from build123d import *

# Parameters (mm, degrees)
F0_R     = 9
F1_DEPTH = 5
F2_R     = 4.15
F3_DEPTH = 1.5
F4_R     = 2.65
F5_DEPTH = 5.001


with BuildPart() as f1:
    # F0 (on Front) → F1 (new body)
    with BuildSketch(Plane.XZ):
        Circle(F0_R)
    extrude(amount=F1_DEPTH)

    # F2 (on face) → F3 (cut)
    with BuildSketch(Plane(origin=(0, 0, 0), x_dir=(-1, 0, 0), z_dir=(0, 1, 0))):
        Circle(F2_R)
    extrude(amount=-F3_DEPTH, mode=Mode.SUBTRACT)

    # F4 (on face) → F5 (cut, through all)
    with BuildSketch(Plane.XZ.offset(5)):
        Circle(F4_R)
    extrude(amount=-F5_DEPTH, mode=Mode.SUBTRACT)


solid = f1.part
Source: CAD feature listing. Evaluate the final solid. Frame: model axes, mm. A direction names the side the tool comes from. Give positions to 0.01 mm unless a question says otherwise; leave off trailing zeros. Write each loop counter-clockwise with the first axis right and the second up, starting at its lowest first coordinate (ties: lowest second). Pieces come first, ordered by that corner, then holes. Notation, with made-up numbers: M 72.25,-0.5 L 105.25,-0.5 A30 cw 105.25,26.5 Z; hole C 61,-4.75 d10. An arc over 180 degrees is marked long. Return JSON: item names as keys, results as strings. Group by question number.
1) Cut plane D-D, the plane z = 6.5. Output: boundary loops of the cut face in (x, y).
2) Ray query, L1, parallel to Z at x = 0, y = -4; L2, parallel to Z at x = 0, y = -1.15; L3, parallel to X at y = -2.8, z = -0.5. Return the intervals inside material, ascending.
3) Cut plane A-A, the plane z = 0. Output: boundary loops of the cut face in (x, y), then the cut area to 3 significant figures.
4) Cut plane B-B, the plane x = 0. Output: boundary loops of the cut face in (y, z), then the cut area to 3 significant figures.
5) Cut plane C-C, the plane y = -0.5. Output: boundary loops of the cut face in (x, z).
6) Draft query along Z for faces 1 (the face through (-1.172, -2.465, 8.923)), 2 (the face through (2, 0, -4)), 3 (the face through (0, -1.5, -3)). Return one class per face: released by +Z, released by -Z, zero draft, split by the parting line, or undercut.
7) Set-up query: faces 4 (the face through (2, -5, -2)), 5 (the face through (0.9, -0.74, -4.05)). Return all of +Z, -Z, +X, -X, +Y, -Y with unobstructed straight access to the full face (end or side cutting, diameter ignored); none if empty.
8) First-contact query: pin 1 Ø5 at (x, z) = (0, 0) entering from -Y; pin 2 Ø2 at (y, z) = (-1, -5.5) entering from +X; pin 3 Ø2 at (x, z) = (-2.5, -1.5) entering from +Y; pin 4 Ø1.5 at (y, z) = (-3.5, 4.5) entering from -X. Flat tips, straight axial feed; report the tip coordinate or a pass-through.
Data:
{
 "1": {"outline": "M -6.22,-5 L 6.22,-5 L 6.22,0 L -6.22,0 Z"},
 "2": {"L1": "z = -9 to -2.65, 2.65 to 9", "L2": "z = -9 to -4.15, 4.15 to 9", "L3": "x = -8.99 to -2.6, 2.6 to 8.99"},
 "3": {"outline": "M -9,-5 L -2.65,-5 L -2.65,-1.5 L -4.15,-1.5 L -4.15,0 L -9,0 Z; M 2.65,-5 L 9,-5 L 9,0 L 4.15,0 L 4.15,-1.5 L 2.65,-1.5 Z", "area": "59.0 mm²"},
 "4": {"outline": "M -5,-9 L 0,-9 L 0,-4.15 L -1.5,-4.15 L -1.5,-2.65 L -5,-2.65 Z; M -5,2.65 L -1.5,2.65 L -1.5,4.15 L 0,4.15 L 0,9 L -5,9 Z", "area": "59.0 mm²"},
 "5": {"outline": "C 0,0 d18; hole C 0,0 d8.3"},
 "6": {"face 1": "split by the parting line", "face 2": "zero draft", "face 3": "undercut"},
 "7": {"face 4": "+Z, -Z, +X, -X, -Y", "face 5": "+Y"},
 "8": {"pin 1": "passes through", "pin 2": "stops at x = 7.79", "pin 3": "stops at y = -1.5", "pin 4": "stops at x = -8.18"}
}
